```python
from build123d import *

# Parameters (mm, degrees)
SKETCH1_W           = 28
SKETCH1_H           = 15.5
BOSS_EXTRUDE1_DEPTH = 4
SKETCH2_R           = 1.25
CUT_EXTRUDE1_DEPTH  = 4
SKETCH3_R           = 2.25
CUT_EXTRUDE2_DEPTH  = 3
SKETCH4_W           = 4.5
SKETCH4_H           = 4.5
CUT_EXTRUDE3_DEPTH  = 1.6
SKETCH5_W           = 4.5
SKETCH5_H           = 1.5
CUT_EXTRUDE4_DEPTH  = 4
SKETCH6_W           = 4.5
SKETCH6_H           = 4.25
CUT_EXTRUDE5_DEPTH  = 1.2
SKETCH7_R           = 2.25
CUT_EXTRUDE6_DEPTH  = 10


with BuildPart() as part:
    # Sketch1 → Boss-Extrude1 (new body)
    with BuildSketch(Plane.XY):
        with Locations((14, -7.75)):
            Rectangle(SKETCH1_W, SKETCH1_H)
    extrude(amount=BOSS_EXTRUDE1_DEPTH)

    # Sketch2 → Cut-Extrude1 (cut)
    with BuildSketch(Plane.XY.offset(4)):
        with Locations((12, -5)):
            Circle(SKETCH2_R)
        with Locations((24, -5)):
            Circle(SKETCH2_R)
    extrude(amount=-CUT_EXTRUDE1_DEPTH, mode=Mode.SUBTRACT)

    # Sketch3 → Cut-Extrude2 (cut)
    with BuildSketch(Plane.XY.offset(4)):
        with Locations((12, -5)):
            Circle(SKETCH3_R)
        with Locations((24, -5)):
            Circle(SKETCH3_R)
    extrude(amount=-CUT_EXTRUDE2_DEPTH, mode=Mode.SUBTRACT)

    # Sketch4 → Cut-Extrude3 (cut)
    with BuildSketch(Plane.XY.offset(4)):
        with Locations((7, -2)):
            Rectangle(SKETCH4_W, SKETCH4_H)
    extrude(amount=-CUT_EXTRUDE3_DEPTH, mode=Mode.SUBTRACT)

    # Sketch5 → Cut-Extrude4 (cut)
    with BuildSketch(Plane.XY.offset(2.4)):
        with Locations((7, -3.5)):
            Rectangle(SKETCH5_W, SKETCH5_H)
    extrude(amount=-CUT_EXTRUDE4_DEPTH, mode=Mode.SUBTRACT)

    # Sketch6 → Cut-Extrude5 (cut)
    with BuildSketch(Plane(origin=(0, 0, 0), x_dir=(-1, 0, 0), z_dir=(0, 0, -1))):
        with Locations((-7, -2.125)):
            Rectangle(SKETCH6_W, SKETCH6_H)
    extrude(amount=-CUT_EXTRUDE5_DEPTH, mode=Mode.SUBTRACT)

    # Sketch7 → Cut-Extrude6 (cut)
    with BuildSketch(Plane.XY.offset(4)):
        with Locations((24, -5)):
            Circle(SKETCH7_R)
    extrude(amount=-CUT_EXTRUDE6_DEPTH, mode=Mode.SUBTRACT)


solid = part.part
```
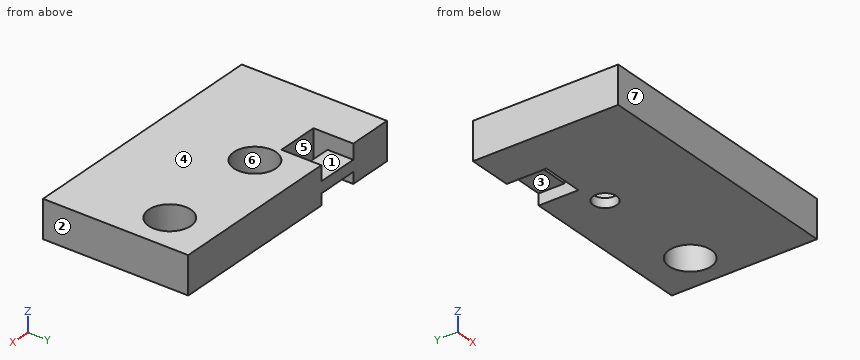
Input: part model. Units: mm. Frame: model coordinates. Face numbers are marked on the shaded views. A direction names the side the tool comes from. Coordinates: 2 decimals unless noted, no trailing zeros. Write each loop counter-clockwise with the first axis right and the second up, starting at its lowest first coordinate (ties: lowest second). Pieces come first, ordered by that corner, then holes.
1) Section C-C on z = 1.95. Output: boundary loops of the cut face in (x, y).
2) Set-up query: the marked faces 5, 6 and 7. Return all of +Z, -Z, +X, -X, +Y, -Y with unobstructed straight access to the full face (end or side cutting, diameter ignored); none if empty.
3) Material intervals for line 1 along Y through (x, z) = (24, 2.6); line 2 along Y through (x, z) = (12, 0.85); line 3 along X through (y, z) = (-5.5, 2), sorted ascending.
4) Pin query (flat end, axial travel): pin 1 Ø2 at (x, y) = (12, -5.5) entering from +Z; pin 2 Ø3 at (x, y) = (7.5, -1.5) entering from +Z. Return the tip coordinate at first contact, or that it passes through.
5) Section B-B on y = -5. Output: boundary loops of the cut face in (x, z).
6) Section D-D on y = -0.75. Output: boundary loops of the cut face in (x, z), and give its area (3 significant figures).
7) Section A-A on x = 12. Output: boundary loops of the cut face in (y, z).
8) Mould query, pull axis X, two halves, no side actions, for the marked faces 1, 2, 3 and 4. Classes: pulls with the +X half, pulls with the -X half, needs draft (parallel to the pull), parting line crosses it, or undercut.
Check result:
1. outline: (0, -15.5) - (28, -15.5) - (28, 0) - (0, 0) - close; hole (4.75, -4.25) - (9.25, -4.25) - (9.25, -2.75) - (4.75, -2.75) - close; hole circle Ø4.5 at (12, -5); hole circle Ø4.5 at (24, -5)
2. face 5: +Z, -Z
2. face 6: +Z
2. face 7: +Z, -Z, +X, -X, -Y
3. line 1: y = -15.5 to -7.25, -2.75 to 0
3. line 2: y = -15.5 to -6.25, -3.75 to 0
3. line 3: x = 0 to 9.81, 14.19 to 21.81, 26.19 to 28
4. pin 1: stops at z = 1
4. pin 2: stops at z = 2.4
5. outline: (0, 0) - (10.75, 0) - (10.75, 1) - (9.75, 1) - (9.75, 4) - (0, 4) - close; (13.25, 0) - (21.75, 0) - (21.75, 4) - (14.25, 4) - (14.25, 1) - (13.25, 1) - close; (26.25, 0) - (28, 0) - (28, 4) - (26.25, 4) - close
6. outline: (0, 0) - (4.75, 0) - (4.75, 1.2) - (9.25, 1.2) - (9.25, 0) - (28, 0) - (28, 4) - (9.25, 4) - (9.25, 2.4) - (4.75, 2.4) - (4.75, 4) - (0, 4) - close
6. area: 99.4 mm2
7. outline: (-15.5, 0) - (-6.25, 0) - (-6.25, 1) - (-7.25, 1) - (-7.25, 4) - (-15.5, 4) - close; (-3.75, 0) - (0, 0) - (0, 4) - (-2.75, 4) - (-2.75, 1) - (-3.75, 1) - close
8. face 1: undercut
8. face 2: pulls with the +X half
8. face 3: undercut
8. face 4: needs draft
